Here's how the part is built. I have some questions about the finished solid (model axes, mm). Face numbers are marked on the shaded views. A direction names the side the tool comes from. Coordinates: 2 decimals unless noted, no trailing zeros. Write each loop counter-clockwise with the first axis right and the second up, starting at its lowest first coordinate (ties: lowest second). Pieces come first, ordered by that corner, then holes.
(1) For pin 1 Ø4 at (x, y) = (1, -43.5) entering from -Z; pin 2 Ø6 at (y, z) = (-20.5, 3.5) entering from -X, each with a flat end and sliding along its axis, tell me the tip position at first contact or that it passes through.
(2) Which directions (+Z, -Z, +X, -X, +Y, -Y) give clear straight access to the entire face, cutting with the end or side of a thin tool? Please do the marked faces 1 and 2.
(3) Please list where these lines run through material, in increasing order: probe 1 along Y at (x, z) = (-4.75, 2); probe 2 along X at (y, z) = (-60.5, 2.25); probe 3 along X at (y, z) = (-57.5, -4).
(4) Imagine slicing it at A-A, the plane y = -12.5. List the corners of the cut face in (x, z) for me, plus the area to 3 significant figures.
Autodesk Inventor part; units mm, degrees
ref_plane "YZ Plane" through (0, 0, 0) normal (1, 0, 0) x (0, 1, 0)
ref_plane "XZ Plane" through (0, 0, 0) normal (0, 1, 0) x (-1, 0, 0)
ref_plane "XY Plane" through (0, 0, 0) normal (0, 0, 1) x (1, 0, 0)
sketch "Sketch1" plane through (0, 0, 0) normal (0, 1, 0) x (-1, 0, 0)
  line L0 (-2.027, 7.8067) -> (5.7473, 5.6588)
  line L1 (5.7473, 5.6588) -> (7.7743, -2.1479)
  line L2 (7.7743, -2.1479) -> (2.027, -7.8067)
  line L3 (2.027, -7.8067) -> (-5.7473, -5.6588)
  line L4 (-5.7473, -5.6588) -> (-7.7743, 2.1479)
  line L5 (-7.7743, 2.1479) -> (-2.027, 7.8067)
  point P0 (0, 0)
  point P1 (0, 0)
  dimension "d8" = 13.97
extrude "Extrusion1" add sketch "Sketch1" along normal blind 6.35
fillet "Fillet1" radius 0.762 6 edges at (4.9007, 6.35, 4.9773) (6.7608, 6.35, -1.7554) (1.8602, 6.35, -6.7328) (-4.9007, 6.35, -4.9773) (-6.7608, 6.35, 1.7554) (-1.8602, 6.35, 6.7328)
sketch "Sketch2" plane through (0, 0, 0) normal (0, -1, 0) x (1, 0, 0)
  circle A0 centre (0, 0) radius 4.6482
  dimension "d3" = 9.2964
extrude "Extrusion2" add sketch "Sketch2" along normal blind 88.9
thread "Thread1"
properties part number "lagBolt_38" material "Steel, Galvanized"
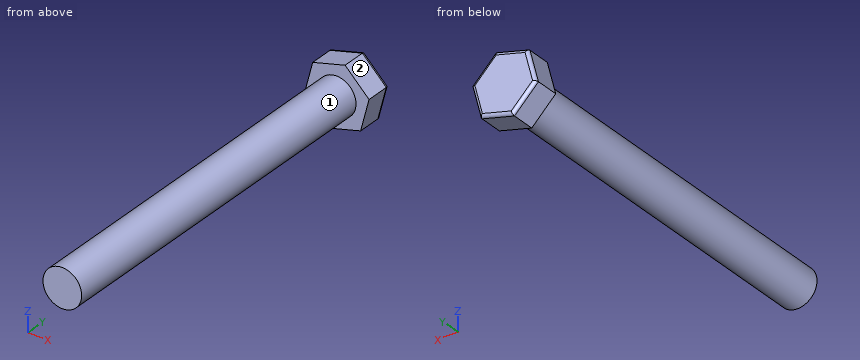
Recorded:
1. pin 1: stops at z = -4.65
1. pin 2: stops at x = -4.62
2. face 1: -Y
2. face 2: +Z, +X, +Y, -Y
3. probe 1: y = 0 to 6.35
3. probe 2: x = -4.07 to 4.07
3. probe 3: x = -2.37 to 2.37
4. outline: circle Ø9.3 at (0, 0)
4. area: 67.9 mm2
